Study the drawing (mm; zero at the part's minimum x, y, z) and answer. Round coordinates to 2 decimals unless told otherwise and drop trailing zeros. Write each loop counter-clockwise with the first axis right and the second up, starting at its lowest first coordinate (ties: lowest second). Pieces come first, ordered by that corner, then holes.
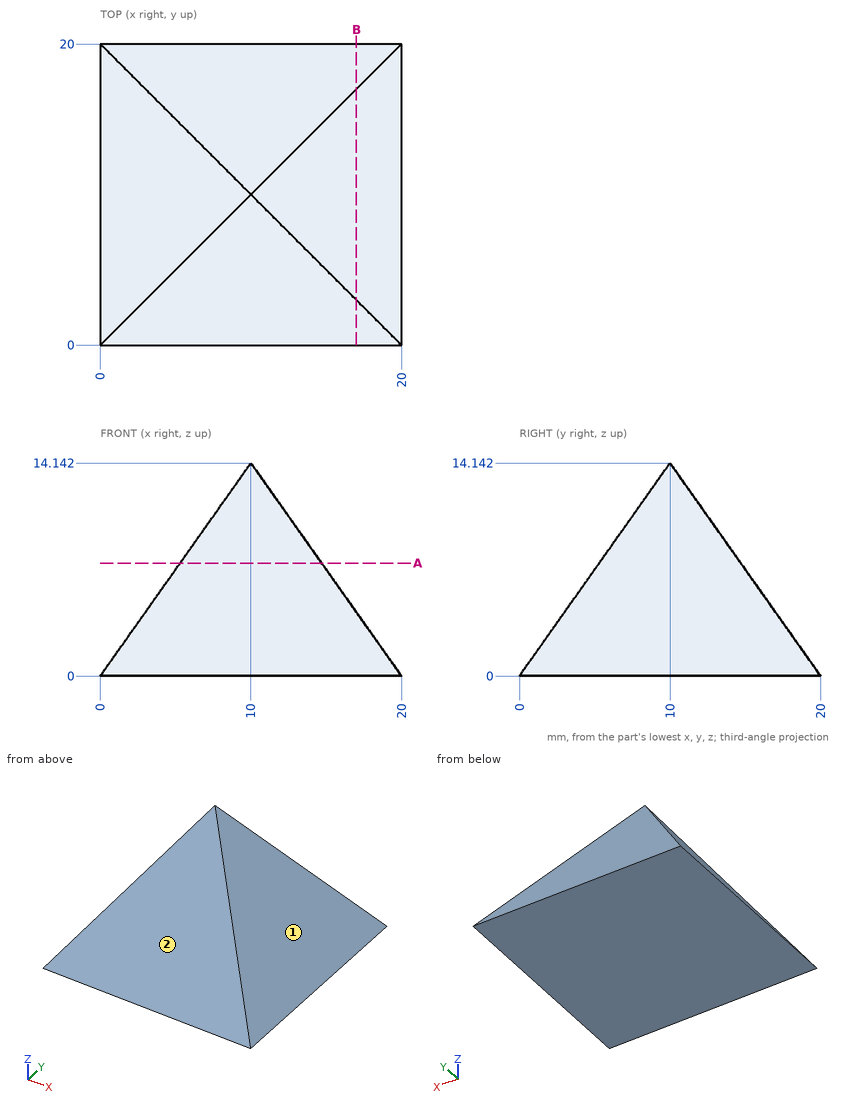
1. Given pin 1 (1 mm diameter, centred on y = 14.5, z = 4.5, fed in from +X); pin 2 (3 mm diameter, centred on x = 12, z = 9.5, fed in from +Y), each flat-ended and moving along its own axis, determine where each tip first touches the part or whether it passes through.
Geometry says:
pin 1: stops at x = 17.17
pin 2: stops at y = 14.34
2. Straight lines are drawn through the part: line 1 along Z through (x, y) = (9.5, 16.25); line 2 along Z through (x, y) = (6.5, 15.25); line 3 along Y through (x, z) = (16.5, 1.25). For each, find the intervals that lie inside material, in ascending order.
Geometry says:
line 1: z = 0 to 5.3
line 2: z = 0 to 6.72
line 3: y = 0.88 to 19.12
3. Section B-B on x = 17 is taken. Determine the outline of the cut face in (y, z).
Geometry says:
outline: (0, 0) - (20, 0) - (17, 4.24) - (3, 4.24) - close
4. For a pull along X with two mould halves and no side action, classify the marked faces 1 and 2 as released by +X, released by -X, zero draft, split by the parting line, or undercut.
Geometry says:
face 1: released by +X
face 2: zero draft
5. Section A-A on z = 7.5 is taken. Determine the outline of the cut face in (x, y), plus the area to 3 significant figures.
Geometry says:
outline: (5.3, 5.3) - (14.7, 5.3) - (14.7, 14.7) - (5.3, 14.7) - close
area: 88.2 mm2
